from build123d import *

# Parameters (mm, degrees)
SKETCH3_W          = 35
SKETCH3_H          = 2.5
CHAMFER1_SIZE      = 0.75
CUT_EXTRUDE1_DEPTH = 1.96
SKETCH9_R          = 1.732050808
CUT_EXTRUDE2_DEPTH = 1.96
CUT_EXTRUDE2_DRAFT = -45


with BuildPart() as part:
    # Sketch3 → Revolve1 (revolve)
    with BuildSketch(Plane(origin=(0, 0, 0), x_dir=(0, 0, -1), z_dir=(1, 0, 0))):
        with Locations((0, 1.25)):
            Rectangle(SKETCH3_W, SKETCH3_H)
    revolve(axis=Axis((0, 0, -17.5), (0, 0, 1)))

    # Chamfer1
    chamfer1_edges = [part.edges().sort_by_distance(p)[0] for p in [
        (0, -2.5, -17.5),
    ]]
    chamfer(chamfer1_edges, length=CHAMFER1_SIZE)

    # Sketch6 → Revolve2 (revolve)
    with BuildSketch(Plane(origin=(0, 0, 0), x_dir=(0, 0, -1), z_dir=(1, 0, 0))):
        Polygon((-17.5, 5), (-17.2, 5), (-14.7, 2.5), (-14.7, 0), (-17.5, 0), align=None)
    revolve(axis=Axis((0, 0, -17.5), (0, 0, 1)))

    # Sketch8 → Cut-Extrude1 (cut)
    with BuildSketch(Plane.XY.offset(17.5)):
        Polygon((0, 1.732050808), (-1.5, 0.866025404), (-1.5, -0.866025404), (0, -1.732050808), (1.5, -0.866025404), (1.5, 0.866025404), align=None)
    extrude(amount=-CUT_EXTRUDE1_DEPTH, mode=Mode.SUBTRACT)


with BuildPart() as cut_extrude2_tool:
    # Sketch9 → Cut-Extrude2 (with draft: the straight prism first)
    with BuildSketch(Plane.XY.offset(17.5)):
        Circle(SKETCH9_R)
    extrude(amount=-CUT_EXTRUDE2_DEPTH)
    # Cut-Extrude2: the draft: its side faces are tilted about the plane it starts from
    cut_extrude2_sides = [cut_extrude2_tool.faces().sort_by_distance(p)[0] for p in [
        (-1.732050808, 0, 16.52),
    ]]
    draft(cut_extrude2_sides, Plane.XY.offset(17.5), CUT_EXTRUDE2_DRAFT)


with BuildPart() as part_1:
    add(part.part)

    # Cut-Extrude2: cut by cut_extrude2_tool
    add(cut_extrude2_tool.part, mode=Mode.SUBTRACT)


solid = part_1.part
CAD build for the part. Positions are in the model's coordinates, mm. A direction names the side the tool comes from. Round coordinates to 2 decimals unless told otherwise and drop trailing zeros. Write each loop counter-clockwise with the first axis right and the second up, starting at its lowest first coordinate (ties: lowest second). Pieces come first, ordered by that corner, then holes.
(1) Drop flat-ended pins along their axis: P1, Ø2, axis at x = -3.5, y = -3, coming from the -Z side; P2, Ø1.4, axis at y = 0, z = 16, coming from the -X side; P3, Ø6, axis at y = -4, z = 1.5, coming from the +X side. Give the stop position or say it passes through.
(2) Slice it at A-A, the plane y = 0. Write the cut outline in (x, z).
(3) Probe line 1 along Z through (x, y) = (0.25, 0.5); line 2 along Z through (x, y) = (0.5, 3.75); line 3 along X through (y, z) = (-0.25, -6.5). List the from-to ranges inside material, lowest first.
(4) Mould opens along X. For faces 1 (the face through (-0.74, 1.305, 16.534)), 2 (the face through (0, 0, -17.5)), 3 (the face through (1.595, -2.08, 14.821)) say: pulls with the +X half, pulls with the -X half, needs draft (parallel to the pull), parting line crosses it, or undercut.
(5) Slice it at B-B, the plane z = -9. Write the cut outline in (x, y), and give its area (3 significant figures).
(6) 3-axis set-ups, long thin cutter, end or side, ignore diameter. For faces 4 (the face through (-1.5, 0, 17)), 5 (the face through (0, -2, 17.5)), 6 (the face through (2.44, -0.54, -1.25)): which of +Z, -Z, +X, -X, +Y, -Y reach the whole face in a straight line?
From the geometry:
1. P1: stops at z = 15.81
1. P2: stops at x = -4.5
1. P3: stops at x = 2.29
2. outline: (-5, 17.2) - (-2.5, 14.7) - (-2.5, -16.75) - (-1.75, -17.5) - (1.75, -17.5) - (2.5, -16.75) - (2.5, 14.7) - (5, 17.2) - (5, 17.5) - (1.73, 17.5) - (1.5, 17.27) - (1.5, 15.54) - (-1.5, 15.54) - (-1.5, 17.27) - (-1.73, 17.5) - (-5, 17.5) - close
3. line 1: z = -17.5 to 15.54
3. line 2: z = 15.98 to 17.5
3. line 3: x = -2.49 to 2.49
4. face 1: undercut
4. face 2: needs draft
4. face 3: parting line crosses it
5. outline: circle Ø5 at (0, 0)
5. area: 19.6 mm2
6. face 4: +Z
6. face 5: +Z, +X, -X, +Y, -Y
6. face 6: -Z
